Verification items for this drawing (mm, ordinates from the low corner). A direction names the side the tool comes from. Round coordinates to 2 decimals unless told otherwise and drop trailing zeros. Write each loop counter-clockwise with the first axis right and the second up, starting at its lowest first coordinate (ties: lowest second). Pieces come first, ordered by that corner, then holes. Notation, with made-up numbers: (84.25, 17) -> (95.25, 17) arc R30 ccw to (95.25, 46) -> close; hole circle Ø7 at (-28.75, -28.75). An arc over 180 degrees is marked (long way). Put each result on its own line as item: value. Start each with the question number.
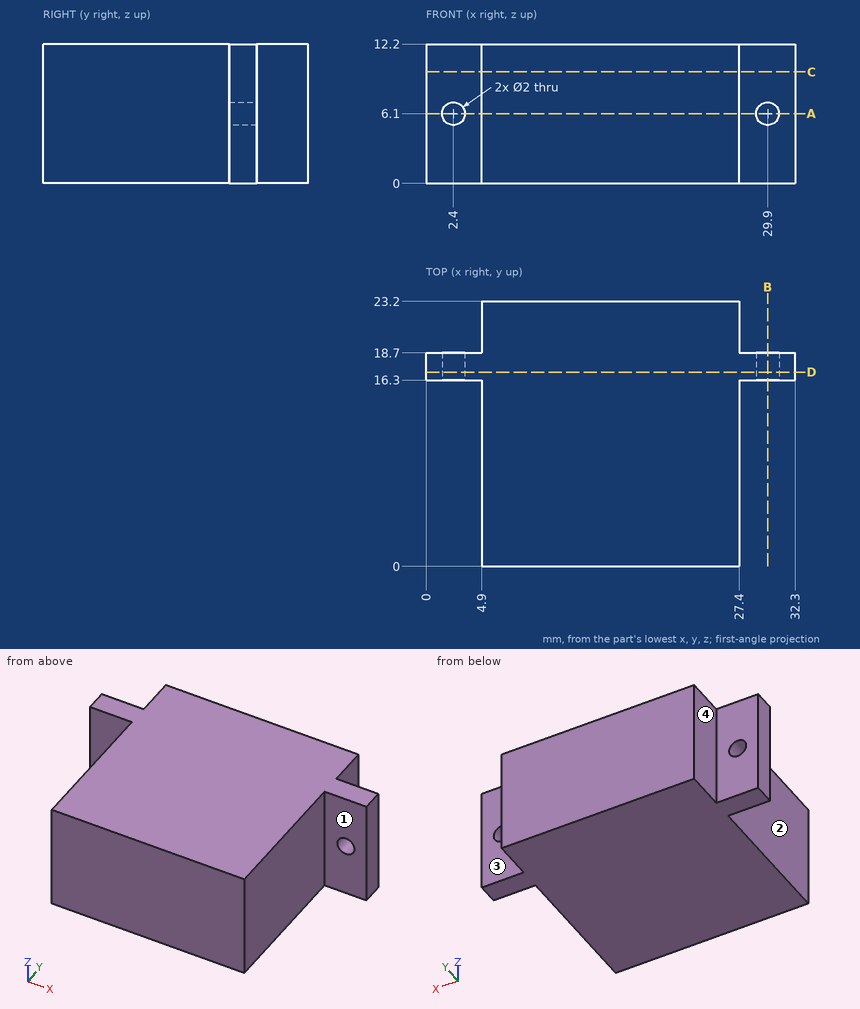
(1) Go/stop test with flat-tipped pins: pin 1 Ø1.6 at (x, z) = (2.4, 6.1) entering from +Y (3 decimals); pin 2 Ø5 at (y, z) = (5.5, 10.5) entering from -X; pin 3 Ø2.5 at (x, z) = (29.9, 6.1) entering from -Y; pin 4 Ø1.3 at (y, z) = (21, 8) entering from +X. Record where each tip stops, or that it passes through.
(2) Sectioned sample at D-D (y = 17). Record the cut outline in (x, z).
(3) Sectioned sample at C-C (z = 9.75). Record the cut outline in (x, y).
(4) Sectioned sample at A-A (z = 6.1). Record the cut outline in (x, y).
(5) Set-up check for the marked faces 1, 2, 3 and 4: record each of +Z, -Z, +X, -X, +Y, -Y from which the full face is reachable in a straight line by a thin tool's end or side.
(6) Material ranges on L1, parallel to X at y = 17.45, z = 6.1; L2, parallel to X at y = 6, z = 4; L3, parallel to Y at x = 1.5, z = 11.25, recorded low to high. Write a range as from..to.
(7) Sectioned sample at B-B (x = 29.9). Record the cut outline in (y, z), and give its area (3 significant figures).
Found:
1. pin 1: through
1. pin 2: x = 4.9
1. pin 3: y = 16.3
1. pin 4: x = 27.4
2. outline: (0, 0) -> (32.3, 0) -> (32.3, 12.2) -> (0, 12.2) -> close; hole circle Ø2 at (2.4, 6.1); hole circle Ø2 at (29.9, 6.1)
3. outline: (0, 16.3) -> (4.9, 16.3) -> (4.9, 0) -> (27.4, 0) -> (27.4, 16.3) -> (32.3, 16.3) -> (32.3, 18.7) -> (27.4, 18.7) -> (27.4, 23.2) -> (4.9, 23.2) -> (4.9, 18.7) -> (0, 18.7) -> close
4. outline: (0, 16.3) -> (1.4, 16.3) -> (1.4, 18.7) -> (0, 18.7) -> close; (3.4, 16.3) -> (4.9, 16.3) -> (4.9, 0) -> (27.4, 0) -> (27.4, 16.3) -> (28.9, 16.3) -> (28.9, 18.7) -> (27.4, 18.7) -> (27.4, 23.2) -> (4.9, 23.2) -> (4.9, 18.7) -> (3.4, 18.7) -> close; (30.9, 16.3) -> (32.3, 16.3) -> (32.3, 18.7) -> (30.9, 18.7) -> close
5. face 1: +Z, -Z, +X, -Y
5. face 2: +Z, -Z, -X, -Y
5. face 3: +Z, -Z, +X, +Y
5. face 4: +Z, -Z, -X, +Y
6. L1: 0..1.4, 3.4..28.9, 30.9..32.3
6. L2: 4.9..27.4
6. L3: 16.3..18.7
7. outline: (16.3, 0) -> (18.7, 0) -> (18.7, 5.1) -> (16.3, 5.1) -> close; (16.3, 7.1) -> (18.7, 7.1) -> (18.7, 12.2) -> (16.3, 12.2) -> close
7. area: 24.5 mm2
